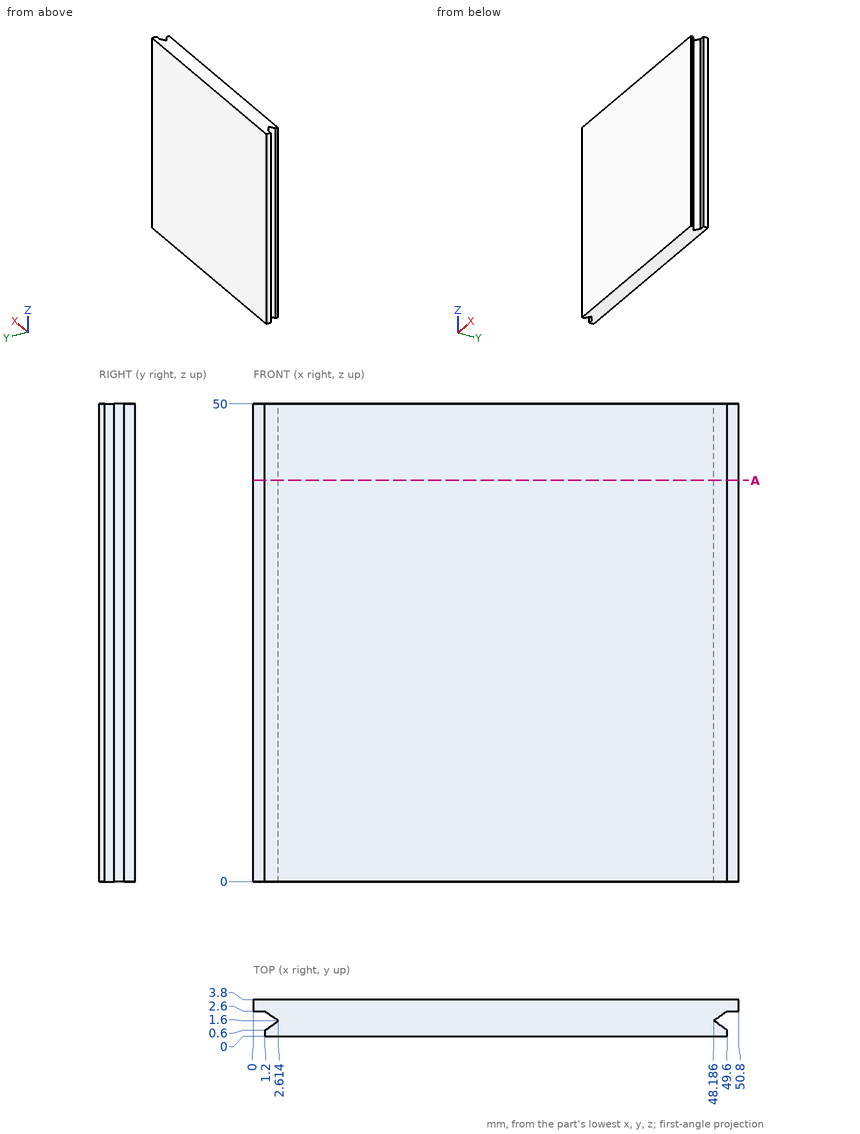
Job drawing, mm, ordinate dimensions from the low corner. One solid piece. Give positions to 0.01 mm unless a question says otherwise; leave off trailing zeros. Write each loop counter-clockwise with the first axis right and the second up, starting at its lowest first coordinate (ties: lowest second). Pieces come first, ordered by that corner, then holes. Notation, with made-up numbers: M 84,60 L 120,60 A17 cw 120,90 Z; hole C 59,48 d1. An arc over 180 degrees is marked long. One line per item, written item: value. Start each with the question number.
Q1. Drop flat-ended pins along their axis: pin 1 Ø0.5 at (y, z) = (0, 23) entering from +X; pin 2 Ø1.3 at (x, z) = (0.5, 13) entering from -Y; pin 3 Ø1.5 at (y, z) = (1, 33) entering from -X. Give the stop position or say it passes through.
Q2. Saw through at A-A, the plane z = 42. Write the cut outline in (x, y), plus the area to 3 significant figures.
Q3. Probe probe 1 along X at (y, z) = (0.4, 39); probe 2 along X at (y, z) = (1.8, 28). List the from-to ranges inside material, lowest first. Write a range as [from, to].
Output values:
1. pin 1: stops at x = 49.6
1. pin 2: stops at y = 2.6
1. pin 3: stops at x = 1.2
2. outline: M 0,2.6 L 1.2,2.6 L 2.61,1.6 L 1.2,0.6 L 1.2,0 L 49.6,0 L 49.6,0.6 L 48.19,1.6 L 49.6,2.6 L 50.8,2.6 L 50.8,3.8 L 0,3.8 Z
2. area: 184 mm²
3. probe 1: x = [1.2, 49.6]
3. probe 2: x = [2.33, 48.47]
